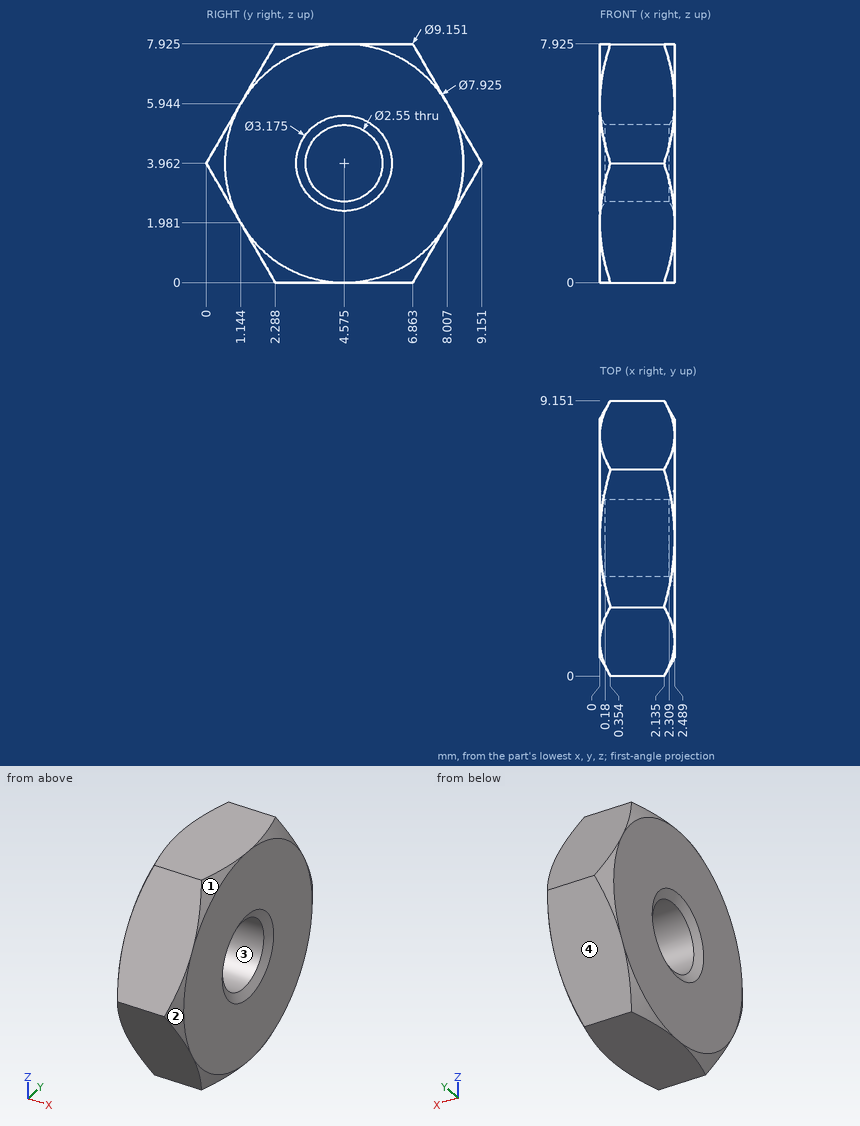
Can you work these out from the drawing? Everything is in mm from the part's minimum corner. Coordinates: 2 decimals unless noted, no trailing zeros.
1) Please list where these lines run through material, in increasing order: line 1 along Z through (x, y) = (0.5, 4.25) (1 decimal); line 2 along Z through (x, y) = (0.7, 5.5) (1 decimal); line 3 along Y through (x, z) = (0.45, 4.25) (1 decimal).
Reported:
line 1: z = 0 to 2.7, 5.2 to 7.9
line 2: z = 0 to 3.1, 4.8 to 7.9
line 3: y = 0.2 to 3.3, 5.8 to 9
2) Thinking about a two-plate mould opening in Z: for the marked faces 1, 2, 3 and 4, which applies, released by +Z, released by -Z, zero draft, split by the parting line, or undercut?
Reported:
face 1: released by +Z
face 2: split by the parting line
face 3: undercut
face 4: released by -Z
3) Will these pins go through, and if not, where does the flat tip stop? pin 1 Ø2 at (y, z) = (6, 4.5) entering from -X; pin 2 Ø1 at (x, y) = (0.5, 1) entering from +Z; pin 3 Ø3 at (y, z) = (4.58, 3.96) entering from +X.
Reported:
pin 1: stops at x = 0
pin 2: stops at z = 6.56
pin 3: stops at x = 2.44
